Read the model definition and answer for the solid it produces. Units are mm, in the model's axes. Face numbers are marked on the shaded views. Round coordinates to 2 decimals unless told otherwise and drop trailing zeros. Order: outer loops, then holes, each group sorted by start corner. A loop starts at its lowest first (then second) coordinate and runs counter-clockwise, first axis right, second up. Notation, with made-up numbers: (-25, -17.5) - (5, -17.5) arc R22 cw to (5, 13.5) - close; hole circle Ø7 at (36.5, -4.75). An arc over 180 degrees is marked (long way). One line per question, with ' | ' between items. Start each with the question number.
1) The part is cut by section A-A, the plane y = 0. Give the vertices of the cut face in (x, z), plus the area to 3 significant figures.
2) The part is cut by section C-C, the plane z = 2.8. Give the vertices of the cut face in (x, y).
3) Straight lines are drawn through the part: line 1 (Y direction, x = 0, z = 4.75); line 2 (Y direction, x = 0.5, z = 2.8); line 3 (X direction, y = -6, z = 3.2). For each, find the intervals that lie inside material, in ascending order. Write a range as from..to.
4) The mould has two halves that part along X. Classify the marked faces 1, 2 and 3: pulls with the +X half, pulls with the -X half, needs draft (parallel to the pull), parting line crosses it, or undercut.
5) Flat-ended cylindrical pins translate along their axes: pin 1 (3 mm diameter, centred on x = 21.22, y = -12.25, fed in from +Z); pin 2 (1 mm diameter, centred on x = -8, z = 2.5, fed in from -Y); pin 3 (1.5 mm diameter, centred on x = -21.22, y = -12.25, fed in from -Z); pin 4 (1.5 mm diameter, centred on y = 5, z = 4.5, fed in from +X). Find the tip coordinate at first contact, or state that the pin passes through.
6) The part is cut by section B-B, the plane x = 5. Give the vertices of the cut face in (y, z).
7) The part is cut by section D-D, the plane y = -12.25. Give the vertices of the cut face in (x, z).
from build123d import *

# Parameters (mm, degrees)
SKETCH_1_R      = 28
SKETCH_1_R_2    = 1.25
SKETCH_1_R_3    = 21.75
EXTRUDE_1_DEPTH = 6


with BuildPart() as part:
    # 草图1 → 凸台-拉伸1 (new body)
    with BuildSketch(Plane.XY):
        Circle(SKETCH_1_R)
        with Locations((0, 24.5)):
            Circle(SKETCH_1_R_2, mode=Mode.SUBTRACT)
        Circle(SKETCH_1_R_3, mode=Mode.SUBTRACT)
        with Locations((21.217622393, 12.25)):
            Circle(SKETCH_1_R_2, mode=Mode.SUBTRACT)
        with Locations((21.217622393, -12.25)):
            Circle(SKETCH_1_R_2, mode=Mode.SUBTRACT)
        with Locations((0, -24.5)):
            Circle(SKETCH_1_R_2, mode=Mode.SUBTRACT)
        with Locations((-21.217622393, -12.25)):
            Circle(SKETCH_1_R_2, mode=Mode.SUBTRACT)
        with Locations((-21.217622393, 12.25)):
            Circle(SKETCH_1_R_2, mode=Mode.SUBTRACT)
    extrude(amount=EXTRUDE_1_DEPTH)


solid = part.part
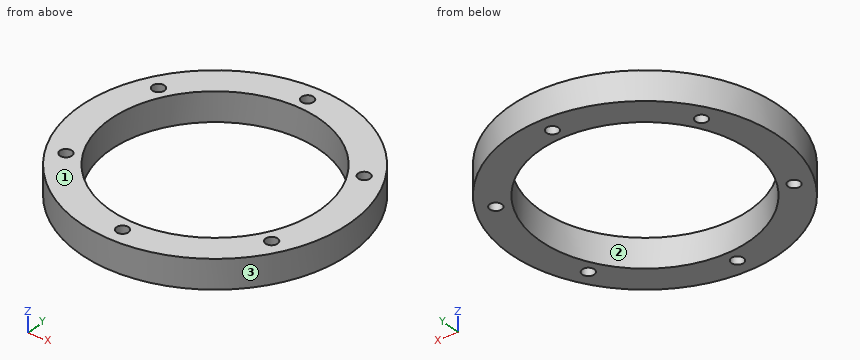
Values:
1) outline: (-28, 0) - (-21.75, 0) - (-21.75, 6) - (-28, 6) - close; (21.75, 0) - (28, 0) - (28, 6) - (21.75, 6) - close | area: 75.0 mm^2
2) outline: circle Ø56 at (0, 0); hole circle Ø2.5 at (-21.22, -12.25); hole circle Ø2.5 at (-21.22, 12.25); hole circle Ø43.5 at (0, 0); hole circle Ø2.5 at (0, -24.5); hole circle Ø2.5 at (0, 24.5); hole circle Ø2.5 at (21.22, -12.25); hole circle Ø2.5 at (21.22, 12.25)
3) line 1: y = -28..-25.75, -23.25..-21.75, 21.75..23.25, 25.75..28 | line 2: y = -28..-25.65, -23.35..-21.74, 21.74..23.35, 25.65..28 | line 3: x = -27.35..-20.91, 20.91..27.35
4) face 1: needs draft | face 2: undercut | face 3: parting line crosses it
5) pin 1: stops at z = 6 | pin 2: stops at y = -26.98 | pin 3: passes through | pin 4: stops at x = 27.68
6) outline: (-27.55, 0) - (-21.17, 0) - (-21.17, 6) - (-27.55, 6) - close; (21.17, 0) - (27.55, 0) - (27.55, 6) - (21.17, 6) - close
7) outline: (-25.18, 0) - (-22.47, 0) - (-22.47, 6) - (-25.18, 6) - close; (-19.97, 0) - (-17.97, 0) - (-17.97, 6) - (-19.97, 6) - close; (17.97, 0) - (19.97, 0) - (19.97, 6) - (17.97, 6) - close; (22.47, 0) - (25.18, 0) - (25.18, 6) - (22.47, 6) - close
